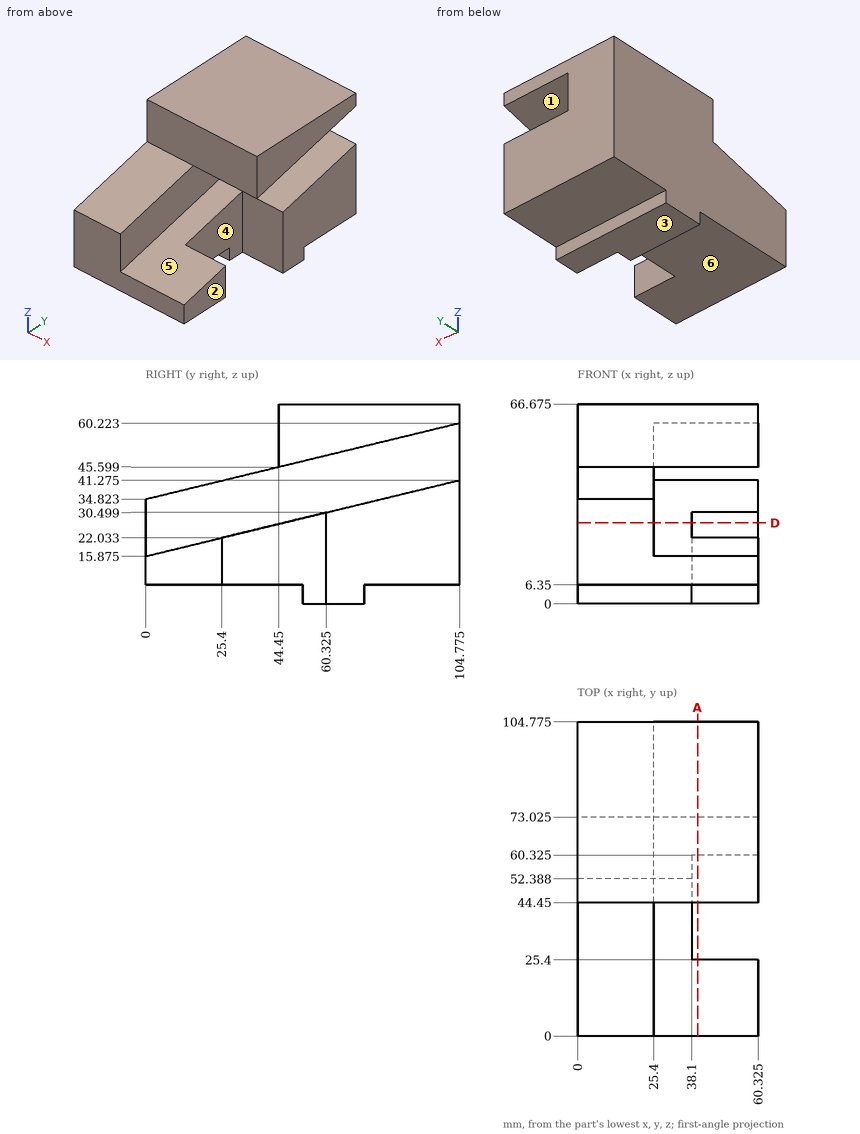
Verification items for this drawing (mm, ordinates from the low corner). A direction names the side the tool comes from. Give positions to 0.01 mm unless a question says otherwise; leave off trailing zeros. Loops run counter-clockwise (first coordinate to the right, second up) from the corner with the lowest first, then second, coordinate; pieces in that order, holes last. Notation, with made-up numbers: M 18.25,18.5 L 55.25,18.5 A25 ccw 55.25,50.5 Z; hole C -17.75,-1 d6. An arc over 180 degrees is marked long. Answer as a JSON object with one key per item and string values. Group by question number.
Q1. Cross-section at A-A on x = 40. Give the number of separate pieces and of enclosed holes in the cut face, then the cut area to 3 significant figures.
Q2. Material ranges on line 1 along Y through (x, z) = (42.5, 7.5) (1 decimal); line 2 along X through (y, z) = (27.5, 30); line 3 along X through (y, z) = (38, 10), recorded low to high. Write a range as [from, to].
Q3. Access from +Z, -Z, +X, -X, +Y, -Y to the whole of each face (thin tool, end or side, straight path). Record for the marked faces 4, 5 and 6.
Q4. Cross-section at D-D on z = 27. Record the cut outline in (x, y) (1 decimal), then the cut area to 3 significant figures.
Q5. Release check for a two-part mould opening along Z. For the marked faces 1, 2 and 3 record: released by +Z, released by -Z, zero draft, split by the parting line, or undercut.
Q6. Go/stop test with flat-tipped pins: P1, Ø2, axis at y = 52.5, z = 12.5, coming from the +X side; P2, Ø5, axis at x = 42.5, z = 11.5, coming from the -Y side; P3, Ø5, axis at x = 19.5, y = 32, coming from the +Z side; P4, Ø10.5, axis at x = 43.5, z = 61, coming from the -Y side. Record where each tip stops, or that it passes through.
Evaluation:
{
 "1": {"separate pieces": "3", "enclosed holes": "0", "area": "2,540 mm2"},
 "2": {"line 1": "y = [0, 25.4], [60.3, 104.8]", "line 2": "x = [0, 25.4]", "line 3": "x = [0, 38.1]"},
 "3": {"face 4": "-Z, +X", "face 5": "+X, -Y", "face 6": "-Z, +X, -X, -Y"},
 "4": {"outline": "M 0,0 L 25.4,0 L 25.4,45.9 L 38.1,45.9 L 38.1,60.3 L 60.3,60.3 L 60.3,104.8 L 0,104.8 Z", "area": "4,400 mm2"},
 "5": {"face 1": "undercut", "face 2": "zero draft", "face 3": "released by -Z"},
 "6": {"P1": "stops at x = 38.1", "P2": "stops at y = 0", "P3": "stops at z = 43.19", "P4": "stops at y = 44.45"}
}
